Geometry check sheet. Reference: drawing and pictorial views, mm from the part's lowest x, y, z. A direction names the side the tool comes from. Give positions to 0.01 mm unless a question says otherwise; leave off trailing zeros. Loops run counter-clockwise (first coordinate to the right, second up) from the corner with the lowest first, then second, coordinate; pieces in that order, holes last. Notation, with made-up numbers: (-3, 44) -> (17, 44) arc R25 cw to (17, 70) -> close; hole circle Ø5 at (64, 51). An arc over 180 degrees is marked (long way). Write each question's results on one line, items separated by ' | '. Start each with the question number.
1. Cross-section at B-B on y = 6.5. Record the boundary of the cut face in (x, z).
2. Cross-section at C-C on z = 10. Record the boundary of the cut face in (x, y), and give its area (3 significant figures).
3. Material ranges on L1, parallel to X at y = 4.5, z = 1.75; L2, parallel to Z at x = 5, y = 10.75; L3, parallel to X at y = 5.5, z = 19.75, recorded low to high. Write a range as from..to.
4. Tool access check on the marked faces 1 and 2. Record the directions out of +Z, -Z, +X, -X, +Y, -Y that give a thin tool (end or side, any length) a straight path to the whole face; none if there is none.
5. Cross-section at A-A on z = 20.5. Record the boundary of the cut face in (x, y), and give its area (3 significant figures).
6. Gauge pin test, flat ends, axial feed: pin 1 Ø3 at (x, z) = (3.5, 8) entering from -Y; pin 2 Ø1.5 at (x, z) = (11.5, 18) entering from +Y; pin 3 Ø4 at (x, z) = (8, 8.5) entering from +Y. Record the tip position at first contact, or that the pin passes through.
7. Mould release check, pull along Y, two halves, no side actions. Record for the marked faces 3, 4, 5 and 6: +Y half, -Y half, draft (parallel to the pull), parting line (faces both ways), or undercut.
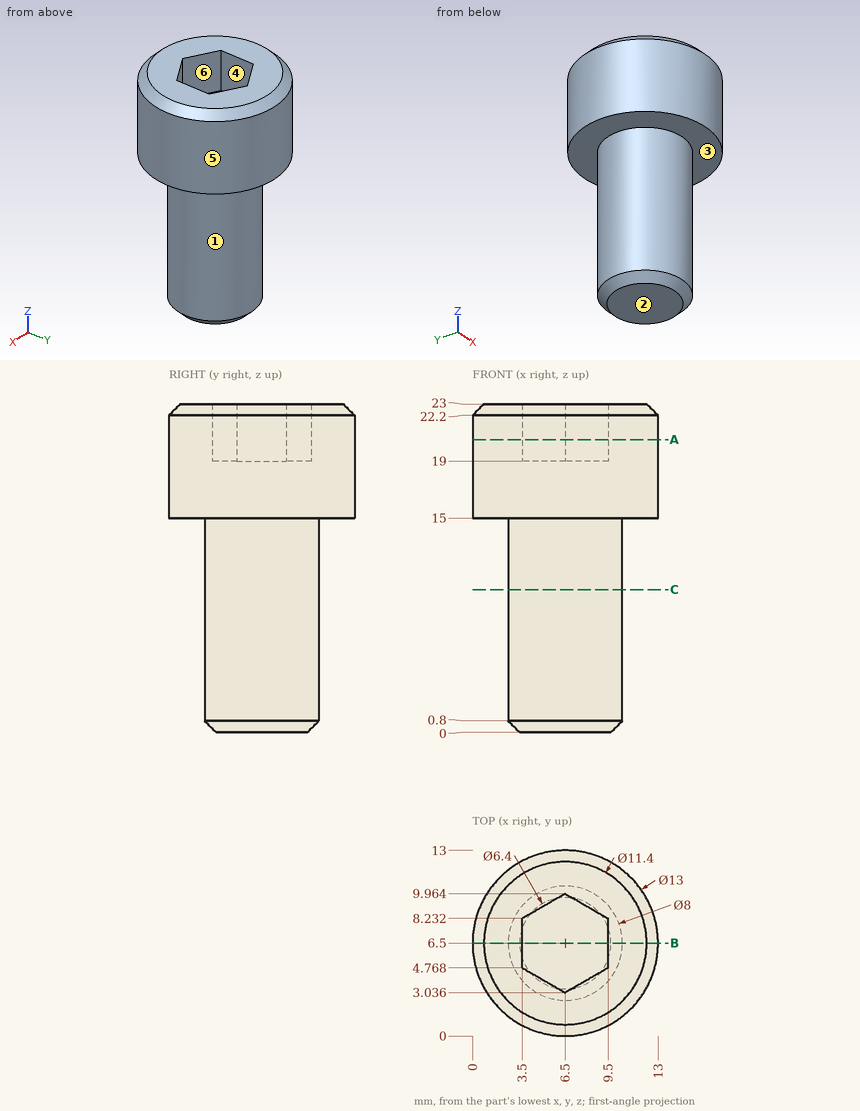
Geometry says:
1) outline: (0, 15) -> (2.5, 15) -> (2.5, 0.8) -> (3.3, 0) -> (9.7, 0) -> (10.5, 0.8) -> (10.5, 15) -> (13, 15) -> (13, 22.2) -> (12.2, 23) -> (9.5, 23) -> (9.5, 19) -> (3.5, 19) -> (3.5, 23) -> (0.8, 23) -> (0, 22.2) -> close
2) outline: circle Ø8 at (6.5, 6.5) | area: 50.3 mm^2
3) L1: 3.04..9.96 | L2: 15..23 | L3: 0.08..3.5, 9.5..12.92
4) face 1: -Z | face 2: -Z, +X, -X, +Y, -Y
5) outline: circle Ø13 at (6.5, 6.5); hole (3.5, 4.77) -> (6.5, 3.04) -> (9.5, 4.77) -> (9.5, 8.23) -> (6.5, 9.96) -> (3.5, 8.23) -> close | area: 102 mm^2
6) pin 1: y = 2.79 | pin 2: y = 11.42 | pin 3: y = 10.5
7) face 3: draft | face 4: undercut | face 5: parting line | face 6: undercut
